Could you check a few things on this model? Use its own coordinates, in mm. Give positions to 0.01 mm unless a question says otherwise; leave off trailing zeros. Loops run counter-clockwise (first coordinate to the right, second up) from the corner with the lowest first, then second, coordinate; pieces in that order, holes last. Notation, with made-up numbers: (-31, 44.5) - (20, 44.5) arc R21 cw to (20, 65.5) - close; hole circle Ø9 at (-37.5, -12). An arc over 180 degrees is marked (long way). Answer in a Markdown table with one row per item. Add a question column.
```python
from build123d import *

# Parameters (mm, degrees)
ESQUISSE1_R        = 1.970435897
ESQUISSE1_R_2      = 1.5
BOSS_EXTRU_1_DEPTH = 4
CONG_1_R           = 15


with BuildPart() as part:
    # Esquisse1 → Boss.-Extru.1 (new body)
    with BuildSketch(Plane.XY):
        with BuildLine():
            Line((55.516963126, 17.477838302), (1.560034717, 18.956280867))
            Line((1.560034717, 18.956280867), (-12.018183396, -33.285157749))
            ThreePointArc((-12.018183396, -33.285157749), (-8.436742053, -39.382146998), (-2.339752804, -35.800705656))
            Line((-2.339752804, -35.800705656), (9.237508154, 8.74216165))
            Line((9.237508154, 8.74216165), (55.243061715, 7.481590105))
            ThreePointArc((55.243061715, 7.481590105), (60.378136519, 12.342763498), (55.516963126, 17.477838302))
        make_face()
        with Locations((5.534972738, 13.003723761)):
            Circle(ESQUISSE1_R, mode=Mode.SUBTRACT)
        with Locations((-7.1789681, -34.542931702)):
            Circle(ESQUISSE1_R_2, mode=Mode.SUBTRACT)
        with Locations((55.380012421, 12.479714203)):
            Circle(ESQUISSE1_R_2, mode=Mode.SUBTRACT)
    extrude(amount=BOSS_EXTRU_1_DEPTH)

    # Congé1
    cong_1_edges = [part.edges().sort_by_distance(p)[0] for p in [
        (1.560034717, 18.956280867, 2),
    ]]
    fillet(cong_1_edges, radius=CONG_1_R)


solid = part.part
```
(1) For pin 1 Ø2.5 at (x, y) = (55.38, 12.48) entering from -Z; pin 2 Ø1 at (x, z) = (5, 1.5) entering from +Y; pin 3 Ø4 at (x, y) = (-7.18, -34.54) entering from -Z; pin 4 Ø1.5 at (y, z) = (-20, 1.5) entering from -X, each with a flat end and sliding along its axis, tell me the tip position at first contact or that it passes through.
(2) We'd pull the mould along X, two halves only. Please class faces 1 (the flat face through (8, 5, 4)), 2 (the flat face through (-6.656, -12.654, 1.972)), 3 (the cylindrical face through (-7.374, -33.056, 1.972)), 4 (the cylindrical face through (5.11, 11.08, 1.97)): pulls with the +X half, pulls with the -X half, needs draft (parallel to the pull), parting line crosses it, or undercut.
(3) Please list where these lines run through material, in increasing order: line 1 (X direction, y = -24, z = 1); line 2 (Y direction, x = 45, z = 3); line 3 (X direction, y = 6, z = 3.25).
(4) I want a section at B-B on y = -26. Please give me the cut outline in (x, z).
(5) I want a section at A-A on z = 2.95. Please give me the cut outline in (x, y), then the cut area to 3 significant figures.
(6) I want a section at C-C on x = 47. Please give me the cut outline in (y, z), then the cut area to 3 significant figures.
Reported:
| question | item | result |
|---|---|---|
| 1 | pin 1 | through |
| 1 | pin 2 | y = 16.58 |
| 1 | pin 3 | z = 0 |
| 1 | pin 4 | x = -8.76 |
| 2 | face 1 | needs draft |
| 2 | face 2 | pulls with the -X half |
| 2 | face 3 | undercut |
| 2 | face 4 | undercut |
| 3 | line 1 | -9.6 to 0.73 |
| 3 | line 2 | 7.76 to 17.77 |
| 3 | line 3 | -1.81 to 8.52 |
| 4 | outline | (-10.12, 0) - (0.21, 0) - (0.21, 4) - (-10.12, 4) - close |
| 5 | outline | (-12.02, -33.29) arc R5 ccw to (-2.34, -35.8) - (9.24, 8.74) - (55.24, 7.48) arc R5 ccw to (55.52, 17.48) - (13.49, 18.63) arc R15 ccw to (-1.44, 7.41) - close; hole circle Ø3 at (-7.18, -34.54); hole circle Ø3.94 at (5.53, 13); hole circle Ø3 at (55.38, 12.48) |
| 5 | area | 1,020 mm² |
| 6 | outline | (7.71, 0) - (17.71, 0) - (17.71, 4) - (7.71, 4) - close |
| 6 | area | 40.0 mm² |
